from build123d import *

# Parameters (mm, degrees)
F3_R     = 16.51
F4_DEPTH = 6.35


with BuildPart() as f1:
    # F0 (on Front) → F1 (revolve)
    with BuildSketch(Plane.XZ):
        Polygon((-13.589, 26.797), (-13.589, 68.58), (-16.256, 68.58), (-17.78, 62.738), (-16.51, 62.738), (-17.78, 56.896), (-16.51, 56.896), (-17.78, 51.054), (-16.51, 51.054), (-17.78, 45.212), (-16.51, 45.212), (-16.51, 0), (-11.7983, 0), (-11.7983, 26.797), align=None)
    revolve(axis=Axis((0, 0, 34.29), (0, 0, 1)))

    # F3 (on offset) → F4 (join)
    with BuildSketch(Plane.XY.offset(30.988)):
        Polygon((19.05, 10.9985226281), (0, 21.9970452561), (-19.05, 10.9985226281), (-19.05, -10.9985226281), (0, -21.9970452561), (19.05, -10.9985226281), align=None)
        Circle(F3_R, mode=Mode.SUBTRACT)
    extrude(amount=-F4_DEPTH)

    # F6 (on Front) → F7 (revolve)
    with BuildSketch(Plane.XZ):
        Polygon((-16.51, 24.638), (-17.018, 24.638), (-16.51, 19.7591881188), align=None)
    revolve(axis=Axis((0, 0, 12.319), (0, 0, 1)))

    # F8 (on Front) → F9 (revolve, cut)
    with BuildSketch(Plane.XZ):
        Polygon((-14.4526, 0), (-16.51, 19.7591881188), (-16.51, 0), align=None)
    revolve(axis=Axis((0, 0, 12.319), (0, 0, 1)), mode=Mode.SUBTRACT)


solid = f1.part
Part model, mm, in its own coordinate system. A direction names the side the tool comes from. Coordinates: 2 decimals unless noted, no trailing zeros. Loops run counter-clockwise (first coordinate to the right, second up) from the corner with the lowest first, then second, coordinate; pieces in that order, holes last. Notation, with made-up numbers: (-19.75, 88.25) - (-12.75, 88.25) arc R10 ccw to (-12.75, 99.25) - close; hole circle Ø5 at (22.25, 67.25). An arc over 180 degrees is marked (long way). Write each question's results on one line, items separated by ' | '. Start each with the question number.
Q1. Which spindle directions (+Z, -Z, +X, -X, +Y, -Y) get a long thin tool onto all of the face, cutting with end or side? Do faces 1 (the flat face through (9.66, 16.42, 27.86)), 2 (the flat face through (0, -12, 26.797)), 3 (the conical face through (-15.823, -4.983, 56.531)). Say none if no direction does.
Q2. Drop flat-ended pins along their axis: pin 1 Ø1.5 at (y, z) = (6, 15) entering from +X; pin 2 Ø13.5 at (x, y) = (6, -2.5) entering from +Z; pin 3 Ø10 at (y, z) = (-4.5, 61) entering from +X. Give the stop position or say it passes through.
Q3. Probe line 1 along X through (y, z) = (0, 44.5); line 2 along Y through (x, z) = (0, 17.25). List the from-to ranges inside material, lowest first.
Q4. Two-plate mould, pull along X, no slides. Class faces 4 (the flat face through (-5.7, -16.2, 24.638)), 5 (the flat face through (19.05, 0, 28)), 6 (the cylindrical face through (2.558, 11.518, 13.586)): +X half, -X half, draft (parallel to the pull), parting line (faces both ways), or undercut.
Q5. Slice it at A-A on z = 7. Give the cut face in (x, y).
Q6. Slice it at C-C on z = 17. Give the cut face in (x, y), and give its area (3 significant figures).
Q7. Slice it at B-B on y = 19.5. Give the cut face in (x, z) (3 decimals), and give its area (3 significant figures).
Answer:
1) face 1: +Z, -Z, +X, +Y | face 2: +Z | face 3: none
2) pin 1: stops at x = 15.14 | pin 2: stops at z = 26.8 | pin 3: stops at x = 17.78
3) line 1: x = -16.51 to -13.59, 13.59 to 16.51 | line 2: y = -16.25 to -11.8, 11.8 to 16.25
4) face 4: draft | face 5: +X half | face 6: undercut
5) outline: circle Ø30.36 at (0, 0); hole circle Ø23.6 at (0, 0)
6) outline: circle Ø32.45 at (0, 0); hole circle Ø23.6 at (0, 0) | area: 389 mm2
7) outline: (-4.325, 24.638) - (4.325, 24.638) - (4.325, 30.988) - (-4.325, 30.988) - close | area: 54.9 mm2
